Input: dimensioned drawing with shaded views. Units: mm. Origin: part minimum x, y, z. A direction names the side the tool comes from. Give positions to 0.01 mm unless a question says otherwise; leave off trailing zeros. Loops run counter-clockwise (first coordinate to the right, second up) from the corner with the lowest first, then second, coordinate; pieces in that order, holes last. Notation, with made-up numbers: M -36.75,65 L -12.75,65 A13 cw -12.75,71 Z; hole C 58,-17 d10. An arc over 180 degrees is marked long. Answer in a Markdown table with one row per item.
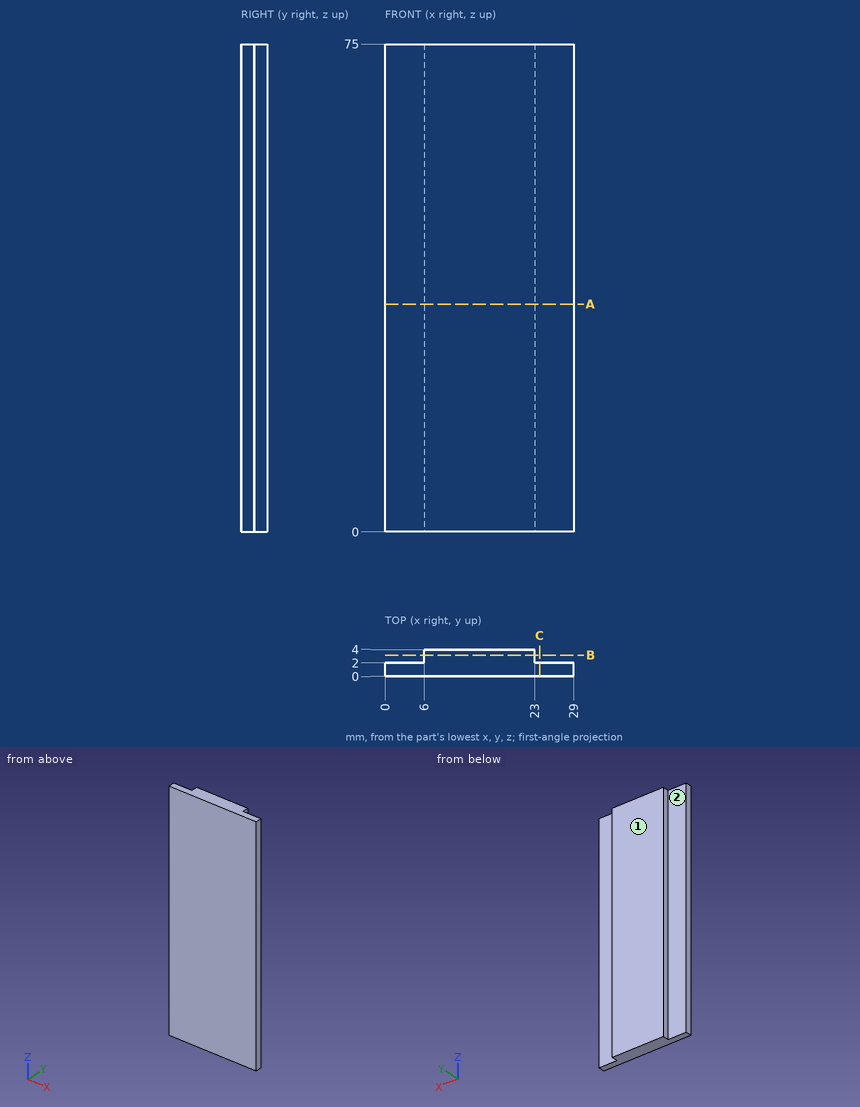
Q1. Section query A-A (z = 35). Output: boundary loops of the cut face in (x, y).
Values follow:
| item | result |
|---|---|
| outline | M 0,0 L 29,0 L 29,2 L 23,2 L 23,4 L 6,4 L 6,2 L 0,2 Z |
Q2. Section query B-B (y = 3.2). Output: boundary loops of the cut face in (x, z), plus the area to 4 significant figures.
Values follow:
| item | result |
|---|---|
| outline | M 6,0 L 23,0 L 23,75 L 6,75 Z |
| area | 1,275 mm^2 |
Q3. Reachability of the marked faces 1 and 2 from +Z, -Z, +X, -X, +Y, -Y: full face, straight path, thin tool, end or side. Return the list, or none.
Values follow:
| item | result |
|---|---|
| face 1 | +Z, -Z, +X, -X, +Y |
| face 2 | +Z, -Z, -X, +Y |
Q4. Section query C-C (x = 23.75). Output: boundary loops of the cut face in (y, z).
Values follow:
| item | result |
|---|---|
| outline | M 0,0 L 2,0 L 2,75 L 0,75 Z |
Q5. Contact query for flat-ended pins moving along their axis: pin 1 Ø3 at (x, z) = (2.5, 53) entering from +Y; pin 2 Ø0.6 at (y, z) = (2.5, 44) entering from +X. Output: stop coordinate, or through.
Values follow:
| item | result |
|---|---|
| pin 1 | y = 2 |
| pin 2 | x = 23 |
Q6. Ray query, probe 1 along Y at (x, z) = (27.5, 66); probe 2 along X at (y, z) = (2.4, 17). Return the intervals inside material, ascending. Write a range as from..to.
Values follow:
| item | result |
|---|---|
| probe 1 | 0..2 |
| probe 2 | 6..23 |
